Part model, mm, in its own coordinate system. Face numbers are marked on the shaded views. A direction names the side the tool comes from. Coordinates: 2 decimals unless noted, no trailing zeros. Order: outer loops, then holes, each group sorted by start corner. A loop starts at its lowest first (then second) coordinate and runs counter-clockwise, first axis right, second up.
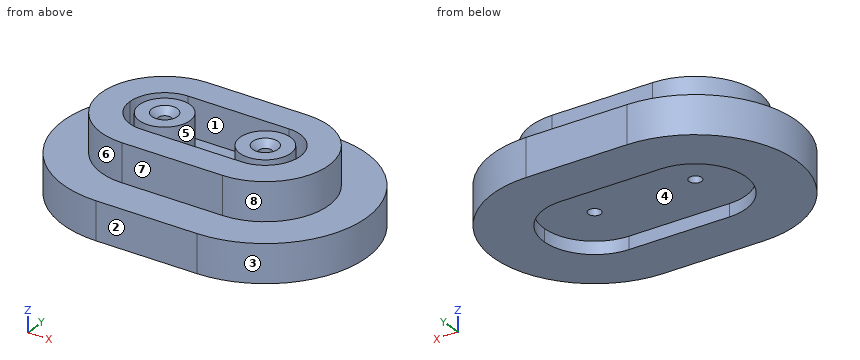
from build123d import *

# Parameters (mm, degrees)
F0_R           = 50.8
F0_R_2         = 12.7
F1_DEPTH       = 76.2
F2_DEPTH       = 152.4
F3_DEPTH       = 152.4
F4_DEPTH       = 25.4
F5_START       = 25.4
F5_DEPTH       = 127
F7_D           = 25.4
F7_CSINK_D     = 50.8
F7_CSINK_ANGLE = 90


# Not quite as in the source:
# - a feature names something its author has since deleted; it is built from what else it names


with BuildPart() as f1:
    # F0 (on Top) → F1 (new body)
    with BuildSketch(Plane.XY):
        with BuildLine():
            ThreePointArc((0, 0), (59.5159020629, -143.6840979371), (203.2, -203.2))
            Line((203.2, -203.2), (406.4, -203.2))
            ThreePointArc((406.4, -203.2), (550.0840979371, -143.6840979371), (609.6, 0))
            ThreePointArc((609.6, 0), (550.0840979371, 143.6840979371), (406.4, 203.2))
            Line((406.4, 203.2), (203.2, 203.2))
            ThreePointArc((203.2, 203.2), (59.5159020629, 143.6840979371), (0, 0))
        make_face()
        with BuildLine():
            Line((406.4, -127), (203.2, -127))
            ThreePointArc((203.2, -127), (113.3974387893, -89.8025612107), (76.2, 0))
            ThreePointArc((76.2, 0), (113.3974387893, 89.8025612107), (203.2, 127))
            Line((203.2, 127), (406.4, 127))
            ThreePointArc((406.4, 127), (496.2025612107, 89.8025612107), (533.4, 0))
            ThreePointArc((533.4, 0), (496.2025612107, -89.8025612107), (406.4, -127))
        make_face(mode=Mode.SUBTRACT)
        with BuildLine():
            ThreePointArc((76.2, 0), (113.3974387893, -89.8025612107), (203.2, -127))
            Line((203.2, -127), (406.4, -127))
            ThreePointArc((406.4, -127), (496.2025612107, -89.8025612107), (533.4, 0))
            ThreePointArc((533.4, 0), (496.2025612107, 89.8025612107), (406.4, 127))
            Line((406.4, 127), (203.2, 127))
            ThreePointArc((203.2, 127), (113.3974387893, 89.8025612107), (76.2, 0))
        make_face()
        with BuildLine():
            Line((406.4, -101.6), (203.2, -101.6))
            ThreePointArc((203.2, -101.6), (131.3579510314, -71.8420489686), (101.6, 0))
            ThreePointArc((101.6, 0), (131.3579510314, 71.8420489686), (203.2, 101.6))
            Line((203.2, 101.6), (406.4, 101.6))
            ThreePointArc((406.4, 101.6), (478.2420489686, 71.8420489686), (508, 0))
            ThreePointArc((508, 0), (478.2420489686, -71.8420489686), (406.4, -101.6))
        make_face(mode=Mode.SUBTRACT)
        with BuildLine():
            ThreePointArc((101.6, 0), (131.3579510314, -71.8420489686), (203.2, -101.6))
            Line((203.2, -101.6), (406.4, -101.6))
            ThreePointArc((406.4, -101.6), (478.2420489686, -71.8420489686), (508, 0))
            ThreePointArc((508, 0), (478.2420489686, 71.8420489686), (406.4, 101.6))
            Line((406.4, 101.6), (203.2, 101.6))
            ThreePointArc((203.2, 101.6), (131.3579510314, 71.8420489686), (101.6, 0))
        make_face()
        with BuildLine():
            ThreePointArc((476.25, 0), (455.7914086659, -49.3914086659), (406.4, -69.85))
            Line((406.4, -69.85), (203.2, -69.85))
            ThreePointArc((203.2, -69.85), (153.8085913341, -49.3914086659), (133.35, 0))
            ThreePointArc((133.35, 0), (153.8085913341, 49.3914086659), (203.2, 69.85))
            Line((203.2, 69.85), (406.4, 69.85))
            ThreePointArc((406.4, 69.85), (455.7914086659, 49.3914086659), (476.25, 0))
        make_face(mode=Mode.SUBTRACT)
        with BuildLine():
            Line((203.2, -69.85), (406.4, -69.85))
            ThreePointArc((406.4, -69.85), (455.7914086659, -49.3914086659), (476.25, 0))
            ThreePointArc((476.25, 0), (455.7914086659, 49.3914086659), (406.4, 69.85))
            Line((406.4, 69.85), (203.2, 69.85))
            ThreePointArc((203.2, 69.85), (153.8085913341, 49.3914086659), (133.35, 0))
            ThreePointArc((133.35, 0), (153.8085913341, -49.3914086659), (203.2, -69.85))
        make_face()
        with Locations((203.2, 0)):
            Circle(F0_R, mode=Mode.SUBTRACT)
        with Locations((406.4, 0)):
            Circle(F0_R, mode=Mode.SUBTRACT)
        with Locations((406.4, 0)):
            Circle(F0_R)
        with Locations((406.4, 0)):
            Circle(F0_R_2, mode=Mode.SUBTRACT)
        with Locations((203.2, 0)):
            Circle(F0_R)
        with Locations((203.2, 0)):
            Circle(F0_R_2, mode=Mode.SUBTRACT)
    extrude(amount=F1_DEPTH)

    # F0 (on Top) → F2 (join)
    with BuildSketch(Plane.XY):
        with BuildLine():
            ThreePointArc((76.2, 0), (113.3974387893, -89.8025612107), (203.2, -127))
            Line((203.2, -127), (406.4, -127))
            ThreePointArc((406.4, -127), (496.2025612107, -89.8025612107), (533.4, 0))
            ThreePointArc((533.4, 0), (496.2025612107, 89.8025612107), (406.4, 127))
            Line((406.4, 127), (203.2, 127))
            ThreePointArc((203.2, 127), (113.3974387893, 89.8025612107), (76.2, 0))
        make_face()
        with BuildLine():
            Line((406.4, -101.6), (203.2, -101.6))
            ThreePointArc((203.2, -101.6), (131.3579510314, -71.8420489686), (101.6, 0))
            ThreePointArc((101.6, 0), (131.3579510314, 71.8420489686), (203.2, 101.6))
            Line((203.2, 101.6), (406.4, 101.6))
            ThreePointArc((406.4, 101.6), (478.2420489686, 71.8420489686), (508, 0))
            ThreePointArc((508, 0), (478.2420489686, -71.8420489686), (406.4, -101.6))
        make_face(mode=Mode.SUBTRACT)
    extrude(amount=F2_DEPTH)

    # F0 (on Top) → F3 (join)
    with BuildSketch(Plane.XY):
        with Locations((203.2, 0)):
            Circle(F0_R)
        with Locations((203.2, 0)):
            Circle(F0_R_2, mode=Mode.SUBTRACT)
        with Locations((406.4, 0)):
            Circle(F0_R)
        with Locations((406.4, 0)):
            Circle(F0_R_2, mode=Mode.SUBTRACT)
        with Locations((203.2, 0)):
            Circle(F0_R_2)
        with Locations((406.4, 0)):
            Circle(F0_R_2)
    extrude(amount=F3_DEPTH)

    # F0 (on Top) → F4 (cut)
    with BuildSketch(Plane.XY):
        with BuildLine():
            ThreePointArc((101.6, 0), (131.3579510314, -71.8420489686), (203.2, -101.6))
            Line((203.2, -101.6), (406.4, -101.6))
            ThreePointArc((406.4, -101.6), (478.2420489686, -71.8420489686), (508, 0))
            ThreePointArc((508, 0), (478.2420489686, 71.8420489686), (406.4, 101.6))
            Line((406.4, 101.6), (203.2, 101.6))
            ThreePointArc((203.2, 101.6), (131.3579510314, 71.8420489686), (101.6, 0))
        make_face()
        with BuildLine():
            ThreePointArc((476.25, 0), (455.7914086659, -49.3914086659), (406.4, -69.85))
            Line((406.4, -69.85), (203.2, -69.85))
            ThreePointArc((203.2, -69.85), (153.8085913341, -49.3914086659), (133.35, 0))
            ThreePointArc((133.35, 0), (153.8085913341, 49.3914086659), (203.2, 69.85))
            Line((203.2, 69.85), (406.4, 69.85))
            ThreePointArc((406.4, 69.85), (455.7914086659, 49.3914086659), (476.25, 0))
        make_face(mode=Mode.SUBTRACT)
        with BuildLine():
            Line((203.2, -69.85), (406.4, -69.85))
            ThreePointArc((406.4, -69.85), (455.7914086659, -49.3914086659), (476.25, 0))
            ThreePointArc((476.25, 0), (455.7914086659, 49.3914086659), (406.4, 69.85))
            Line((406.4, 69.85), (203.2, 69.85))
            ThreePointArc((203.2, 69.85), (153.8085913341, 49.3914086659), (133.35, 0))
            ThreePointArc((133.35, 0), (153.8085913341, -49.3914086659), (203.2, -69.85))
        make_face()
        with Locations((203.2, 0)):
            Circle(F0_R, mode=Mode.SUBTRACT)
        with Locations((406.4, 0)):
            Circle(F0_R, mode=Mode.SUBTRACT)
        with Locations((203.2, 0)):
            Circle(F0_R)
        with Locations((203.2, 0)):
            Circle(F0_R_2, mode=Mode.SUBTRACT)
        with Locations((406.4, 0)):
            Circle(F0_R)
        with Locations((406.4, 0)):
            Circle(F0_R_2, mode=Mode.SUBTRACT)
    extrude(amount=F4_DEPTH, mode=Mode.SUBTRACT)

    # F0 (on Top) → F5 (join)
    with BuildSketch(Plane.XY.offset(F5_START)):
        with BuildLine():
            ThreePointArc((101.6, 0), (131.3579510314, -71.8420489686), (203.2, -101.6))
            Line((203.2, -101.6), (406.4, -101.6))
            ThreePointArc((406.4, -101.6), (478.2420489686, -71.8420489686), (508, 0))
            ThreePointArc((508, 0), (478.2420489686, 71.8420489686), (406.4, 101.6))
            Line((406.4, 101.6), (203.2, 101.6))
            ThreePointArc((203.2, 101.6), (131.3579510314, 71.8420489686), (101.6, 0))
        make_face()
        with BuildLine():
            ThreePointArc((476.25, 0), (455.7914086659, -49.3914086659), (406.4, -69.85))
            Line((406.4, -69.85), (203.2, -69.85))
            ThreePointArc((203.2, -69.85), (153.8085913341, -49.3914086659), (133.35, 0))
            ThreePointArc((133.35, 0), (153.8085913341, 49.3914086659), (203.2, 69.85))
            Line((203.2, 69.85), (406.4, 69.85))
            ThreePointArc((406.4, 69.85), (455.7914086659, 49.3914086659), (476.25, 0))
        make_face(mode=Mode.SUBTRACT)
    extrude(amount=F5_DEPTH)

    # F7 (through all)
    with Locations(Plane.XY.offset(152.4)):
        with Locations((203.2, 0), (406.4, 0)):
            CounterSinkHole(F7_D / 2, F7_CSINK_D / 2, counter_sink_angle=F7_CSINK_ANGLE)


solid = f1.part
Q1. Mould opens along X. For the marked faces 1, 2 and 3 say: pulls with the +X half, pulls with the -X half, needs draft (parallel to the pull), parting line crosses it, or undercut.
Results list:
face 1: undercut
face 2: needs draft
face 3: pulls with the +X half
Q2. Pin check, flat tips, straight feed: pin 1 Ø23 at (x, z) = (279.5, 126.5) entering from +Y; pin 2 Ø10 at (x, z) = (521.5, 44) entering from -Y; pin 3 Ø4 at (x, z) = (86.5, 47.5) entering from +Y. Stop position of each tip, or through.
Results list:
pin 1: stops at y = 127
pin 2: stops at y = -170.79
pin 3: stops at y = 167.73
Q3. Which spindle directions (+Z, -Z, +X, -X, +Y, -Y) get a long thin tool onto all of the face, cutting with end or side? Do the marked faces 4, 5, 6, 7 and 8. Say none if no direction does.
Results list:
face 4: -Z
face 5: +Z
face 6: +Z, -X
face 7: +Z, +X, -X, -Y
face 8: +Z, +X
Q4. Cut at B-B on x = 367. Write the cut outline in (y, z), and give its area (3 significant figures).
Results list:
outline: (-203.2, 0) - (-101.6, 0) - (-101.6, 25.4) - (101.6, 25.4) - (101.6, 0) - (203.2, 0) - (203.2, 76.2) - (127, 76.2) - (127, 152.4) - (69.85, 152.4) - (69.85, 76.2) - (32.07, 76.2) - (32.07, 152.4) - (-32.07, 152.4) - (-32.07, 76.2) - (-69.85, 76.2) - (-69.85, 152.4) - (-127, 152.4) - (-127, 76.2) - (-203.2, 76.2) - close
area: 39,400 mm2
Q5. Cut at C-C on y = 90.5. Write the cut outline in (x, z), and give its area (3 significant figures).
Results list:
outline: (21.27, 0) - (157.02, 0) - (157.02, 25.4) - (452.58, 25.4) - (452.58, 0) - (588.33, 0) - (588.33, 76.2) - (495.5, 76.2) - (495.5, 152.4) - (114.1, 152.4) - (114.1, 76.2) - (21.27, 76.2) - close
area: 64,800 mm2
Q6. Cut at D-D on x = 544. Write the cut outline in (y, z).
Results list:
outline: (-149.52, 0) - (149.52, 0) - (149.52, 76.2) - (-149.52, 76.2) - close
Q7. Cut at A-A on z = 92. Write the cut outline in (x, y).
Results list:
outline: circle Ø101.6 at (203.2, 0); (203.2, -127) - (406.4, -127) arc R127 ccw to (406.4, 127) - (203.2, 127) arc R127 ccw to start; circle Ø101.6 at (406.4, 0); hole circle Ø25.4 at (203.2, 0); hole (203.2, -69.85) - (406.4, -69.85) arc R69.85 ccw to (406.4, 69.85) - (203.2, 69.85) arc R69.85 ccw to start; hole circle Ø25.4 at (406.4, 0)
Q8. Wall check: line 1 along Y through (x, z) = (203.2, 113); line 2 along X through (y, z) = (0, 67); line 3 along Y through (x, z) = (406.4, 55). Give the ranges that are in metal, low to high.
Results list:
line 1: y = -127 to -69.85, -50.8 to -12.7, 12.7 to 50.8, 69.85 to 127
line 2: x = 0 to 190.5, 215.9 to 393.7, 419.1 to 609.6
line 3: y = -203.2 to -12.7, 12.7 to 203.2
